Here's how the part is built. I have some questions about the finished solid (model axes, mm). Face numbers are marked on the shaded views. A direction names the side the tool comes from. Coordinates: 2 decimals unless noted, no trailing zeros. Loops run counter-clockwise (first coordinate to the right, second up) from the corner with the lowest first, then second, coordinate; pieces in that order, holes last.
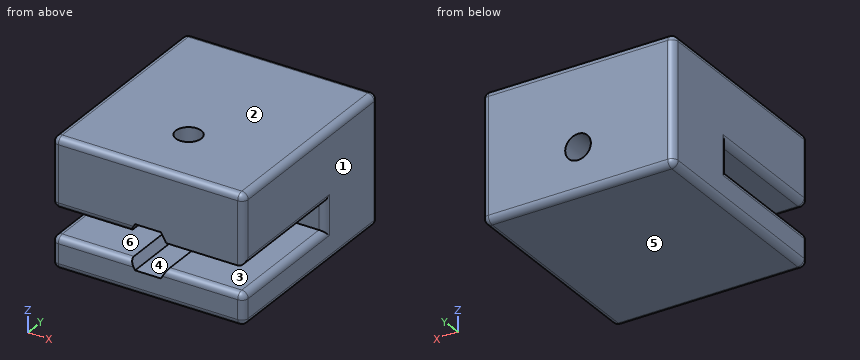
from build123d import *

# Parameters (mm, degrees)
F0_W          = 30
F0_H          = 33
F1_DEPTH      = 20
F2_W          = 20
F2_H          = 4.2
F3_DEPTH      = 30.001
F4_R          = 2
F5_DEPTH      = 5
F5_DEPTH_BACK = 20.001
F6_DEPTH      = 13.001
F7_R          = 2
F8_DEPTH      = 10.801
F9_DEPTH      = 3.5
F10_R         = 1


with BuildPart() as f1:
    # F0 (on Top) → F1 (new body)
    with BuildSketch(Plane.XY):
        Rectangle(F0_W, F0_H)
    extrude(amount=F1_DEPTH)

    # F2 (on face) → F3 (cut, through all)
    with BuildSketch(Plane.YZ.offset(15)):
        with Locations((-6.5, 7.1)):
            Rectangle(F2_W, F2_H)
    extrude(amount=-F3_DEPTH, mode=Mode.SUBTRACT)

    # F4 (on face) → F5 (cut, two sides)
    with BuildSketch(Plane.XZ.offset(-3.5)) as f5_sk:
        Polygon((-2.829016319, 9.2), (2.829016319, 9.2), (2.0207259422, 10.6), (-2.0207259422, 10.6), align=None)
        Polygon((-2.829016319, 5), (2.829016319, 5), (4.0414518843, 7.1), (2.829016319, 9.2), (-2.829016319, 9.2), (-4.0414518843, 7.1), align=None)
        with Locations((0, 7.1)):
            Circle(F4_R, mode=Mode.SUBTRACT)
        Polygon((-2.0207259422, 3.6), (2.0207259422, 3.6), (2.829016319, 5), (-2.829016319, 5), align=None)
    extrude(amount=-F5_DEPTH, mode=Mode.SUBTRACT)
    extrude(f5_sk.sketch, amount=F5_DEPTH_BACK, mode=Mode.SUBTRACT)

    # F6 (cut, through all): a face of the model
    f6_faces = [f1.faces().sort_by_distance(p)[0] for p in [
        (0, 3.5, 7.1),
    ]]
    extrude(f6_faces, amount=-F6_DEPTH, mode=Mode.SUBTRACT)

    # F7 (on face) → F8 (cut, through all)
    with BuildSketch(Plane(origin=(0, 0, 9.2), x_dir=(1, 0, 0), z_dir=(0, 0, -1))):
        with Locations((0, 6.5)):
            Circle(F7_R)
    extrude(amount=-F8_DEPTH, mode=Mode.SUBTRACT)

    # F7 (on face) → F9 (cut)
    with BuildSketch(Plane(origin=(0, 0, 9.2), x_dir=(1, 0, 0), z_dir=(0, 0, -1))):
        Polygon((-4.0414518843, 6.5), (-2.829016319, 4.4), (-2.829016319, 8.6), align=None)
        Polygon((-2.829016319, 8.6), (-2.829016319, 4.4), (-2.0207259422, 3), (2.0207259422, 3), (2.829016319, 4.4), (2.829016319, 8.6), (2.0207259422, 10), (-2.0207259422, 10), align=None)
        with Locations((0, 6.5)):
            Circle(F7_R, mode=Mode.SUBTRACT)
        Polygon((2.829016319, 8.6), (2.829016319, 4.4), (4.0414518843, 6.5), align=None)
    extrude(amount=-F9_DEPTH, mode=Mode.SUBTRACT)

    # F10
    f10_edges = [f1.edges().sort_by_distance(p)[0] for p in [
        (0, 16.5, 0),
        (15, 16.5, 10),
        (0, 16.5, 20),
        (-15, 16.5, 10),
        (-15, 0, 0),
        (0, -16.5, 0),
        (15, 0, 0),
        (-15, 0, 20),
        (0, -16.5, 20),
        (15, 0, 20),
        (-15, -16.5, 2.5),
        (-15, -16.5, 14.6),
        (15, -16.5, 2.5),
        (15, -16.5, 14.6),
        (15, -6.5, 9.2),
        (15, -6.5, 5),
        (8.914508, -16.5, 5),
        (-8.914508, -16.5, 5),
        (-8.914508, -16.5, 9.2),
        (-15, 3.5, 7.1),
        (-15, -6.5, 5),
        (-15, -6.5, 9.2),
        (15, 3.5, 7.1),
    ]]
    fillet(f10_edges, radius=F10_R)


solid = f1.part
Q1. For the marked faces 4, 5 and 6, which set-ups out of +Z, -Z, +X, -X, +Y, -Y let a thin tool reach every point of the face, with its end or its side?
Q2. Will these pins go through, and if not, where does the flat tip stop? P1, Ø5, axis at x = 0, z = 7.1, coming from the -Y side; P2, Ø1.5, axis at x = -4, z = 6, coming from the -Y side.
Q3. We'd pull the mould along Z, two halves only. Please class the marked faces 1, 2 and 3: pulls with the +Z half, pulls with the -Z half, needs draft (parallel to the pull), parting line crosses it, or undercut.
Q4. Suppose I cut it at C-C on z = 8.25. Write out the boundary of the cut face in (x, y), and give its area (3 significant figures).
Q5. Suppose I cut it at B-B on x = 0. Write out the boundary of the cut face in (y, z), and give its area (3 significant figures).
Q6. Suppose I cut it at D-D on x = 12. Write out the boundary of the cut face in (y, z), and give its area (3 significant figures).
Q7. Suppose I cut it at A-A on y = -14. Write out the boundary of the cut face in (x, z), and give its area (3 significant figures).
Q8. Please list where these lines run through material, in increasing order: probe 1 along X at (y, z) = (-6.5, 18.5); probe 2 along Z at (x, y) = (-10.25, -5); probe 3 along X at (y, z) = (-10, 4).
Check values:
1. face 4: -Y
1. face 5: -Z, +X, -X, +Y, -Y
1. face 6: +X, -X, -Y
2. P1: stops at y = 8.5
2. P2: stops at y = 3.5
3. face 1: needs draft
3. face 2: pulls with the +Z half
3. face 3: undercut
4. outline: (-15, 4.5) arc R1 ccw to (-14, 3.5) - (-3.38, 3.5) - (-3.38, 8.5) - (-1.64, 8.5) - (-1.64, 16.5) - (-14, 16.5) arc R1 ccw to (-15, 15.5) - close; (1.64, 8.5) - (3.38, 8.5) - (3.38, 3.5) - (14, 3.5) arc R1 ccw to (15, 4.5) - (15, 15.5) arc R1 ccw to (14, 16.5) - (1.64, 16.5) - close
4. area: 329 mm2
5. outline: (-16.5, 1) arc R1 ccw to (-15.5, 0) - (15.5, 0) arc R1 ccw to (16.5, 1) - (16.5, 5.1) - (8.5, 5.1) - (8.5, 3.6) - (-16.5, 3.6) - close; (-16.5, 10.6) - (-10, 10.6) - (-10, 12.7) - (-8.5, 12.7) - (-8.5, 20) - (-15.5, 20) arc R1 ccw to (-16.5, 19) - close; (-4.5, 12.7) - (-3, 12.7) - (-3, 10.6) - (8.5, 10.6) - (8.5, 9.1) - (16.5, 9.1) - (16.5, 19) arc R1 ccw to (15.5, 20) - (-4.5, 20) - close
5. area: 408 mm2
6. outline: (-16.5, 1) arc R1 ccw to (-15.5, 0) - (15.5, 0) arc R1 ccw to (16.5, 1) - (16.5, 19) arc R1 ccw to (15.5, 20) - (-15.5, 20) arc R1 ccw to (-16.5, 19) - (-16.5, 9.2) - (3.5, 9.2) - (3.5, 5) - (-15.5, 5) arc R1 ccw to (-16.5, 4) - close
6. area: 575 mm2
7. outline: (-15, 1) arc R1 ccw to (-14, 0) - (14, 0) arc R1 ccw to (15, 1) - (15, 4) arc R1 ccw to (14, 5) - (2.83, 5) - (2.02, 3.6) - (-2.02, 3.6) - (-2.83, 5) - (-14, 5) arc R1 ccw to (-15, 4) - close; (-15, 10.2) arc R1 ccw to (-14, 9.2) - (-2.83, 9.2) - (-2.02, 10.6) - (2.02, 10.6) - (2.83, 9.2) - (14, 9.2) arc R1 ccw to (15, 10.2) - (15, 19) arc R1 ccw to (14, 20) - (-14, 20) arc R1 ccw to (-15, 19) - close
7. area: 459 mm2
8. probe 1: x = -15 to -2, 2 to 15
8. probe 2: z = 0 to 5, 9.2 to 20
8. probe 3: x = -15 to -2.25, 2.25 to 15
